Verification items for the finished model (mm, model axes). A direction names the side the tool comes from. Coordinates: 2 decimals unless noted, no trailing zeros. Loops run counter-clockwise (first coordinate to the right, second up) from the corner with the lowest first, then second, coordinate; pieces in that order, holes last. Notation, with made-up numbers: (45.5, -17) -> (50.5, -17) arc R14 ccw to (50.5, -4) -> close; hole circle Ø8 at (-6.75, -3.75). An arc over 180 degrees is marked (long way). Write item = value, one per line.
```python
from build123d import *

# Parameters (mm, degrees)
F3_DEPTH = 15
F4_R     = 15
F5_DEPTH = 141
F7_DEPTH = 10


with BuildPart() as f1:
    # F0 (on Top) → F1 (revolve)
    with BuildSketch(Plane.XY):
        Polygon((0, 19.0511253548), (0, -30.9488746452), (50, -30.9488746452), (50, -10.9488746452), (30, -10.9488746452), (30, 19.0511253548), align=None)
    revolve(axis=Axis((0, -5.9488746452, 0), (0, 1, 0)))

    # F2 (on face) → F3 (cut)
    with BuildSketch(Plane.XZ.offset(30.9488746452)):
        with BuildLine():
            ThreePointArc((6, 49.638694584), (0, 50), (-6, 49.638694584))
            Line((-6, 49.638694584), (-6, -49.638694584))
            ThreePointArc((-6, -49.638694584), (0, -50), (6, -49.638694584))
            Line((6, -49.638694584), (6, 49.638694584))
        make_face()
    extrude(amount=-F3_DEPTH, mode=Mode.SUBTRACT)

    # F4 (on face) → F5 (cut)
    with BuildSketch(Plane(origin=(0, 19.0511253548, 0), x_dir=(-1, 0, 0), z_dir=(0, 1, 0))):
        Circle(F4_R)
    extrude(amount=-F5_DEPTH, mode=Mode.SUBTRACT)

    # F6 (on face) → F7 (cut)
    with BuildSketch(Plane(origin=(0, 19.0511253548, 0), x_dir=(-1, 0, 0), z_dir=(0, 1, 0))):
        with BuildLine():
            Line((3, 14.6969384567), (3, 18))
            Line((3, 18), (-3, 18))
            Line((-3, 18), (-3, 14.6969384567))
            ThreePointArc((-3, 14.6969384567), (0, 15), (3, 14.6969384567))
        make_face()
    extrude(amount=-F7_DEPTH, mode=Mode.SUBTRACT)


solid = f1.part
```
1) Sectioned sample at D-D, the plane z = 23. Record the cut outline in (x, y), plus the area to 3 significant figures.
Ans:
outline = (-44.4, -30.95) -> (-6, -30.95) -> (-6, -15.95) -> (6, -15.95) -> (6, -30.95) -> (44.4, -30.95) -> (44.4, -10.95) -> (19.26, -10.95) -> (19.26, 19.05) -> (-19.26, 19.05) -> (-19.26, -10.95) -> (-44.4, -10.95) -> close
area = 2,750 mm2
2) Sectioned sample at A-A, the plane x = 0. Record the cut outline in (y, z), plus the area to 3 significant figures.
Ans:
outline = (-15.95, -50) -> (-10.95, -50) -> (-10.95, -30) -> (19.05, -30) -> (19.05, -15) -> (-15.95, -15) -> close; (-15.95, 15) -> (9.05, 15) -> (9.05, 18) -> (19.05, 18) -> (19.05, 30) -> (-10.95, 30) -> (-10.95, 50) -> (-15.95, 50) -> close
area = 1,220 mm2
3) Tool access check on faces 4 (the face through (6, 19.051, -14)), 5 (the face through (0, -15.949, -32)), 6 (the face through (3, 14, 16)). Record the directions out of +Z, -Z, +X, -X, +Y, -Y that give a thin tool (end or side, any length) a straight path to the whole face; none if there is none.
Ans:
face_4 = +Z, -Z, +X, -X, +Y
face_5 = +Z, -Z, -Y
face_6 = +Y
4) Sectioned sample at C-C, the plane y = 13. Record the cut outline in (x, z), plus the area to 3 significant figures.
Ans:
outline = circle Ø60 at (0, 0); hole (-3, 14.7) arc R15 ccw (long way) to (3, 14.7) -> (3, 18) -> (-3, 18) -> close
area = 2,100 mm2
5) Depth check by flat-ended pin: pin 1 Ø16.5 at (y, z) = (-21.5, -32.5) entering from -X; pin 2 Ø3.5 at (y, z) = (15.5, 15.5) entering from -X; pin 3 Ø1 at (x, y) = (-21.5, -16) entering from +Z. Enter the tip coordinate at first touch or a pass-through.
Ans:
pin_1 = -43.73
pin_2 = -26.66
pin_3 = 45.38
6) Sectioned sample at B-B, the plane z = 0. Record the cut outline in (x, y), plus the area to 3 significant figures.
Ans:
outline = (-50, -30.95) -> (-15, -30.95) -> (-15, 19.05) -> (-30, 19.05) -> (-30, -10.95) -> (-50, -10.95) -> close; (15, -30.95) -> (50, -30.95) -> (50, -10.95) -> (30, -10.95) -> (30, 19.05) -> (15, 19.05) -> close
area = 2,300 mm2
7) Material ranges on line 1 (X direction, y = 9.5, z = 0); line 2 (Y direction, x = -28.5, z = 22.5), recorded low to high.
Ans:
line_1 = -30 to -15, 15 to 30
line_2 = -30.95 to -10.95
8) Release check for a two-part mould opening along Z. For faces 1 (the face through (47.69, -20.81, -15.02)), 2 (the face through (-28, -30.949, -1)), 3 (the face through (-3, 14, 16)) record: pulls with the +Z half, pulls with the -Z half, needs draft (parallel to the pull), parting line crosses it, or undercut.
Ans:
face_1 = parting line crosses it
face_2 = needs draft
face_3 = undercut
